from build123d import *

# Parameters (mm, degrees)
SKETCH1_R        = 7.9
EXTRUSION2_DEPTH = 19.05
EXTRUSION3_REACH = 24.084
SKETCH2_R        = 5
SKETCH3_R        = 14.25
EXTRUSION4_DEPTH = 5.08
EXTRUSION5_REACH = 29.676
SKETCH4_R        = 5


with BuildPart() as part:
    # Sketch1 → Extrusion2 (new body)
    with BuildSketch(Plane(origin=(0, 5, 0), x_dir=(1, 0, 0), z_dir=(0, 1, 0))):
        with Locations(Location((0, 0, 0), (0, 0, 90))):
            Circle(SKETCH1_R)
    extrude(amount=EXTRUSION2_DEPTH)

    # Sketch2 → Extrusion3 (cut, up to next)
    with BuildSketch(Plane(origin=(0, 24.05, 0), x_dir=(-1, 0, 0), z_dir=(0, 1, 0)), mode=Mode.PRIVATE) as extrusion3_sk1:
        with Locations(Location((0, 0, 0), (0, 0, 90))):
            Circle(SKETCH2_R)
    extrusion3_tool1 = extrude(extrusion3_sk1.sketch, amount=-EXTRUSION3_REACH, mode=Mode.PRIVATE) & part.part
    add(extrusion3_tool1.solids().sort_by_distance((0, 24.05, 0))[0], mode=Mode.SUBTRACT)

    # Sketch3 → Extrusion4 (add)
    with BuildSketch(Plane(origin=(0, 0, 0), x_dir=(-1, 0, 0), z_dir=(0, 1, 0))):
        with Locations(Location((0, 0, 0), (0, 0, 90))):
            Circle(SKETCH3_R)
    extrude(amount=EXTRUSION4_DEPTH)

    # Sketch4 → Extrusion5 (cut, up to next)
    with BuildSketch(Plane(origin=(0, 5.08, 0), x_dir=(-1, 0, 0), z_dir=(0, 1, 0)), mode=Mode.PRIVATE) as extrusion5_sk1:
        with Locations(Location((0, 0, 0), (0, 0, 90))):
            Circle(SKETCH4_R)
    extrusion5_tool1 = extrude(extrusion5_sk1.sketch, amount=-EXTRUSION5_REACH, mode=Mode.PRIVATE) & part.part
    add(extrusion5_tool1.solids().sort_by_distance((0, 5.08, 0))[0], mode=Mode.SUBTRACT)


solid = part.part
Verification items for the finished model (mm, model axes). A direction names the side the tool comes from. Give positions to 0.01 mm unless a question says otherwise; leave off trailing zeros. Write each loop counter-clockwise with the first axis right and the second up, starting at its lowest first coordinate (ties: lowest second). Pieces come first, ordered by that corner, then holes. Notation, with made-up numbers: (43, 20.25) - (54, 20.25) arc R18 ccw to (54, 32.25) - close; hole circle Ø2 at (-28, 82). An arc over 180 degrees is marked (long way). Answer as CSV lines item,"result". Start each with the question number.
1. Sectioned sample at B-B (x = 0). Record the boundary of the cut face in (y, z), then the cut area to 3 significant figures.
2. Draft check along Z on faces 3 (the face through (-6, 5.08, 6)), 4 (the face through (-13.91, 2.5, -3.09)), 5 (the face through (-4.88, 12.19, -1.08)). Enter one of: pulls with the +Z half, pulls with the -Z half, needs draft (parallel to the pull), parting line crosses it, or undercut.
3. Sectioned sample at A-A (z = 0). Record the boundary of the cut face in (x, y).
4. Thickness scan on line 1 (X direction, y = 16, z = 0); line 2 (Z direction, x = -4.5, y = 8.25); line 3 (Y direction, x = 13, z = 0.75). Record the ranges inside material, lowest first.
5. Set-up check for faces 1 (the face through (-6, 0, 0)), 2 (the face through (-5.34, 14.43, 5.82)): record each of +Z, -Z, +X, -X, +Y, -Y from which the full face is reachable in a straight line by a thin tool's end or side.
6. Sectioned sample at C-C (y = 20.75). Record the boundary of the cut face in (x, z).
7. Sectioned sample at D-D (x = 9). Record the boundary of the cut face in (y, z).
8. Depth check by flat-ended pin: pin 1 (2 mm diameter, centred on x = 10, z = 8, fed in from -Y); pin 2 (4 mm diameter, centred on y = 21, z = 4, fed in from +X); pin 3 (6 mm diameter, centred on x = -9.5, z = -6.5, fed in from +Y); pin 4 (6 mm diameter, centred on x = 0, z = 0, fed in from -Y). Enter the tip coordinate at first touch or a pass-through.
Derived:
1,outline,"(0, -14.25) - (5.08, -14.25) - (5.08, -7.9) - (24.05, -7.9) - (24.05, -5) - (0, -5) - close; (0, 5) - (24.05, 5) - (24.05, 7.9) - (5.08, 7.9) - (5.08, 14.25) - (0, 14.25) - close"
1,area,"204 mm²"
2,face 3,"needs draft"
2,face 4,"parting line crosses it"
2,face 5,"undercut"
3,outline,"(-14.25, 0) - (-5, 0) - (-5, 24.05) - (-7.9, 24.05) - (-7.9, 5.08) - (-14.25, 5.08) - close; (5, 0) - (14.25, 0) - (14.25, 5.08) - (7.9, 5.08) - (7.9, 24.05) - (5, 24.05) - close"
4,line 1,"-7.9 to -5, 5 to 7.9"
4,line 2,"-6.49 to -2.18, 2.18 to 6.49"
4,line 3,"0 to 5.08"
5,face 1,"+Z, -Z, +X, -X, -Y"
5,face 2,"+Y"
6,outline,"circle Ø15.8 at (0, 0); hole circle Ø10 at (0, 0)"
7,outline,"(0, -11.05) - (5.08, -11.05) - (5.08, 11.05) - (0, 11.05) - close"
8,pin 1,"y = 0"
8,pin 2,"x = 7.64"
8,pin 3,"y = 5.08"
8,pin 4,"through"
